Verification items for the finished model (mm, model axes). Face numbers are marked on the shaded views. A direction names the side the tool comes from. Give positions to 0.01 mm unless a question says otherwise; leave off trailing zeros. Write each loop counter-clockwise with the first axis right and the second up, starting at its lowest first coordinate (ties: lowest second). Pieces come first, ordered by that corner, then holes. Notation, with made-up numbers: (-35, 24.25) -> (20, 24.25) arc R26 ccw to (20, 60.25) -> close; hole circle Ø9 at (61.5, -15.75). An arc over 180 degrees is marked (long way). Use CSV: the item, a comma, the result in double quotes. Start each with the question number.
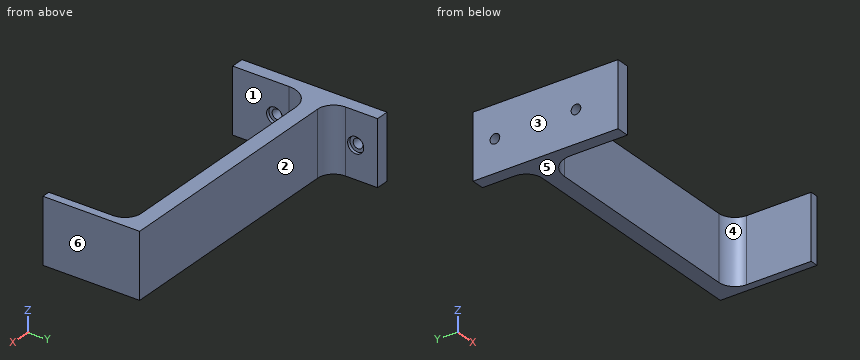
```python
from build123d import *

# Parameters (mm, degrees)
ESQUISSE2_W             = 170
ESQUISSE2_H             = 40
BOSS_EXTRU_1_DEPTH      = 10
ESQUISSE3_W             = 8
ESQUISSE3_H             = 40
BOSS_EXTRU_2_DEPTH      = 50
ESQUISSE4_W             = 5
ESQUISSE4_H             = 40
BOSS_EXTRU_3_DEPTH      = 50
CONG_1_R                = 15
CONG_2_R                = 10
ESQUISSE7_W             = 8
ESQUISSE7_H             = 40
BOSS_EXTRU_4_DEPTH      = 30
CONG_3_R                = 10
ENL_V_MAT_EXTRU_3_REACH = 180.326
ESQUISSE8_R             = 3
ESQUISSE10_R            = 5
ENL_V_MAT_EXTRU_4_DEPTH = 2
ESQUISSE11_R            = 5
ENL_V_MAT_EXTRU_5_DEPTH = 2


with BuildPart() as part:
    # Esquisse2 → Boss.-Extru.1 (new body)
    with BuildSketch(Plane(origin=(0, 0, 0), x_dir=(1, 0, 0), z_dir=(0, 1, 0))):
        Rectangle(ESQUISSE2_W, ESQUISSE2_H)
    extrude(amount=BOSS_EXTRU_1_DEPTH)

    # Esquisse3 → Boss.-Extru.2 (add)
    with BuildSketch(Plane.XZ):
        with Locations((-81, 0)):
            Rectangle(ESQUISSE3_W, ESQUISSE3_H)
    extrude(amount=BOSS_EXTRU_2_DEPTH)

    # Esquisse4 → Boss.-Extru.3 (add)
    with BuildSketch(Plane.XZ):
        with Locations((82.5, 0)):
            Rectangle(ESQUISSE4_W, ESQUISSE4_H)
    extrude(amount=BOSS_EXTRU_3_DEPTH)

    # Congé1
    cong_1_edges = [part.edges().sort_by_distance(p)[0] for p in [
        (-77, 0, 0),
    ]]
    fillet(cong_1_edges, radius=CONG_1_R)

    # Congé2
    cong_2_edges = [part.edges().sort_by_distance(p)[0] for p in [
        (80, 0, 0),
    ]]
    fillet(cong_2_edges, radius=CONG_2_R)

    # Esquisse7 → Boss.-Extru.4 (add)
    with BuildSketch(Plane(origin=(0, 10, 0), x_dir=(1, 0, 0), z_dir=(0, 1, 0))):
        with Locations((-81, 0)):
            Rectangle(ESQUISSE7_W, ESQUISSE7_H)
    extrude(amount=BOSS_EXTRU_4_DEPTH)

    # Congé3
    cong_3_edges = [part.edges().sort_by_distance(p)[0] for p in [
        (-77, 10, 0),
    ]]
    fillet(cong_3_edges, radius=CONG_3_R)

    # Esquisse8 → Enlèv. mat.-Extru.3 (cut, up to next)
    with BuildSketch(Plane.ZY.offset(85), mode=Mode.PRIVATE) as enl_v_mat_extru_3_sk1:
        with Locations((0, 26.38656459)):
            Circle(ESQUISSE8_R)
    enl_v_mat_extru_3_tool1 = extrude(enl_v_mat_extru_3_sk1.sketch, amount=-ENL_V_MAT_EXTRU_3_REACH, mode=Mode.PRIVATE) & part.part
    # Esquisse8 → Enlèv. mat.-Extru.3 (cut, up to next)
    with BuildSketch(Plane.ZY.offset(85), mode=Mode.PRIVATE) as enl_v_mat_extru_3_sk2:
        with Locations((0, -23.907675409)):
            Circle(ESQUISSE8_R)
    enl_v_mat_extru_3_tool2 = extrude(enl_v_mat_extru_3_sk2.sketch, amount=-ENL_V_MAT_EXTRU_3_REACH, mode=Mode.PRIVATE) & part.part
    add(enl_v_mat_extru_3_tool1.solids().sort_by_distance((-85, 26.386565, 0))[0], mode=Mode.SUBTRACT)
    add(enl_v_mat_extru_3_tool2.solids().sort_by_distance((-85, -23.907675, 0))[0], mode=Mode.SUBTRACT)

    # Esquisse10 → Enlèv. mat.-Extru.4 (cut)
    with BuildSketch(Plane(origin=(-77, 0, 0), x_dir=(0, 0, -1), z_dir=(1, 0, 0))):
        with Locations((0, -23.907675409)):
            Circle(ESQUISSE10_R)
    extrude(amount=-ENL_V_MAT_EXTRU_4_DEPTH, mode=Mode.SUBTRACT)

    # Esquisse11 → Enlèv. mat.-Extru.5 (cut)
    with BuildSketch(Plane(origin=(-77, 0, 0), x_dir=(0, 0, -1), z_dir=(1, 0, 0))):
        with Locations((0, 26.38656459)):
            Circle(ESQUISSE11_R)
    extrude(amount=-ENL_V_MAT_EXTRU_5_DEPTH, mode=Mode.SUBTRACT)


solid = part.part
```
(1) Section check C-C on z = -10. Record the cut outline in (x, y), then the cut area to 3 significant figures.
(2) Draft check along X on the marked faces 4, 5 and 6. Enter one of: released by +X, released by -X, zero draft, split by the parting line, or undercut.
(3) Section check B-B on y = -4.5. Record the cut outline in (x, z), then the cut area to 3 significant figures.
(4) Section check D-D on x = -34. Record the cut outline in (y, z).
(5) Section check A-A on z = 0. Give the number of separate pieces and of enclosed holes in the cut face, then the cut area to 3 significant figures.
(6) Thickness scan on line 1 (Y direction, x = -77.65, z = 0); line 2 (Y direction, x = -82, z = 0); line 3 (X direction, y = -18, z = 3). Record the ranges inside material, lowest first. Write a range as from..to.
(7) Set-up check for the marked faces 1, 2 and 3: record each of +Z, -Z, +X, -X, +Y, -Y from which the full face is reachable in a straight line by a thin tool's end or side.
(8) Go/stop test with flat-tipped pins: pin 1 (6 mm diameter, centred on x = 11, z = -9.5, fed in from -Y); pin 2 (3.5 mm diameter, centred on y = 26.39, z = 0, fed in from +X); pin 3 (1 mm diameter, centred on x = 5, z = 7, fed in from +Y); pin 4 (8 mm diameter, centred on y = 28, z = -1, fed in from +X). Record where each tip stops, or that it passes through.
Data:
1,outline,"(-85, -50) -> (-77, -50) -> (-77, -15) arc R15 cw to (-62, 0) -> (70, 0) arc R10 cw to (80, -10) -> (80, -50) -> (85, -50) -> (85, 10) -> (-67, 10) arc R10 cw to (-77, 20) -> (-77, 40) -> (-85, 40) -> close"
1,area,"2,680 mm2"
2,face 4,"undercut"
2,face 5,"zero draft"
2,face 6,"released by +X"
3,outline,"(-85, -20) -> (-72.71, -20) -> (-72.71, 20) -> (-85, 20) -> close; (78.35, -20) -> (85, -20) -> (85, 20) -> (78.35, 20) -> close"
3,area,"757 mm2"
4,outline,"(0, -20) -> (10, -20) -> (10, 20) -> (0, 20) -> close"
5,separate pieces,"3"
5,enclosed holes,"0"
5,area,"2,570 mm2"
6,line 1,"y = -50..-28.91, -18.91..21.39, 31.39..40"
6,line 2,"y = -50..-26.91, -20.91..23.39, 29.39..40"
6,line 3,"x = -85..-77, 80..85"
7,face 1,"+Z, -Z, -Y"
7,face 2,"+Z, -Z, +X, +Y"
7,face 3,"+Z, -Z, -X, +Y, -Y"
8,pin 1,"stops at y = 0"
8,pin 2,"passes through"
8,pin 3,"stops at y = 10"
8,pin 4,"stops at x = -77"
